Check sheet for the modelled part. Datum: model origin and axes. Units: mm. A direction names the side the tool comes from. Give positions to 0.01 mm unless a question says otherwise; leave off trailing zeros. Loops run counter-clockwise (first coordinate to the right, second up) from the corner with the lowest first, then second, coordinate; pieces in that order, holes last. Notation, with made-up numbers: M 69.25,-32.75 L 88.25,-32.75 A20 cw 88.25,-20.75 Z; hole C 64.25,-3 d4. An arc over 180 degrees is marked long. Put each result on its own line as item: value. Start each with the question number.
```python
from build123d import *

# Parameters (mm, degrees)
BOSS_EXTRUDE1_DEPTH = 390
SKETCH2_R           = 2
CUT_EXTRUDE1_DEPTH  = 392.02429592
CUT_EXTRUDE2_DEPTH  = 392.02429592
FILLET1_R           = 5


with BuildPart() as part:
    # Sketch1 → Boss-Extrude1 (new body)
    with BuildSketch(Plane(origin=(0, 0, 0), x_dir=(0, 0, -1), z_dir=(1, 0, 0))):
        Polygon((0, 0), (20, 0), (20, 3.461178467), (3.461178467, 3.461178467), (3.461178467, 20), (0, 20), align=None)
    extrude(amount=BOSS_EXTRUDE1_DEPTH)

    # Sketch2 → Cut-Extrude1 (cut, through all)
    with BuildSketch(Plane.XZ):
        with Locations(Location((195, -10, 0), (0, 0, 270))):
            Circle(SKETCH2_R)
        with Locations(Location((335, -10, 0), (0, 0, 270))):
            Circle(SKETCH2_R)
        with Locations(Location((55, -10, 0), (0, 0, 270))):
            Circle(SKETCH2_R)
        with Locations(Location((383, -10, 0), (0, 0, 270))):
            Circle(SKETCH2_R)
        with Locations(Location((7, -10, 0), (0, 0, 270))):
            Circle(SKETCH2_R)
    extrude(amount=-CUT_EXTRUDE1_DEPTH, mode=Mode.SUBTRACT)

    # Sketch3 → Cut-Extrude2 (cut, through all)
    with BuildSketch(Plane.XY):
        Polygon((0, 7.5), (20, 7.5), (32.5, 20), (0, 20), align=None)
        Polygon((390, 20), (357.5, 20), (370, 7.5), (390, 7.5), align=None)
    extrude(amount=-CUT_EXTRUDE2_DEPTH, mode=Mode.SUBTRACT)

    # Fillet1
    fillet1_edges = [part.edges().sort_by_distance(p)[0] for p in [
        (390, 1.730589234, -20),
        (0, 1.730589234, -20),
    ]]
    fillet(fillet1_edges, radius=FILLET1_R)


solid = part.part
```
Q1. Section check B-B, the plane y = 15.5. Record the cut outline in (x, z).
Q2. Section check A-A, the plane x = 86.5. Record the cut outline in (y, z), then the cut area to 3 significant figures.
Q3. Access from +Z, -Z, +X, -X, +Y, -Y to the whole of each face (thin tool, end or side, straight path). Record for faces 1 (the face through (192, 12, -3.461)), 2 (the face through (363.7, 13.8, -1.7)).
Q4. Thickness scan on line 1 along X through (y, z) = (2.5, -10); line 2 along Z through (x, y) = (335, 2.5); line 3 along Y through (x, z) = (137, -7.5). Record the ranges inside material, lowest first. Write a range as [from, to].
Q5. Depth check by flat-ended pin: P1, Ø3, axis at x = 303.5, z = -9, coming from the +Y side; P2, Ø1, axis at x = 375, z = -2, coming from the +Y side; P3, Ø3, axis at x = 7, z = -10, coming from the +Y side; P4, Ø4, axis at x = 274.5, y = 14, coming from the -Z side. Enter the tip coordinate at first touch or a pass-through.
Found:
1. outline: M 28,-3.46 L 362,-3.46 L 362,0 L 28,0 Z
2. outline: M 0,-20 L 3.46,-20 L 3.46,-3.46 L 20,-3.46 L 20,0 L 0,0 Z
2. area: 126 mm^2
3. face 1: -Z, +X, -X, +Y
3. face 2: +Z, -Z, +X, +Y
4. line 1: x = [0, 5], [9, 53], [57, 193], [197, 333], [337, 381], [385, 390]
4. line 2: z = [-20, -12], [-8, 0]
4. line 3: y = [0, 3.46]
5. P1: stops at y = 3.46
5. P2: stops at y = 7.5
5. P3: passes through
5. P4: stops at z = -3.46
